Input: part model. Units: mm. Frame: model coordinates. Face numbers are marked on the shaded views. A direction names the side the tool comes from. Round coordinates to 2 decimals unless told otherwise and drop trailing zeros. Write each loop counter-clockwise with the first axis right and the second up, starting at its lowest first coordinate (ties: lowest second). Pieces come first, ordered by that corner, then holes. Notation, with made-up numbers: (76, -20) -> (91, -20) arc R22 ccw to (91, -2) -> close; hole circle Ø7 at (-25, 5.5). An arc over 180 degrees is marked (long way). Write item = value, one per line. Start each with the question number.
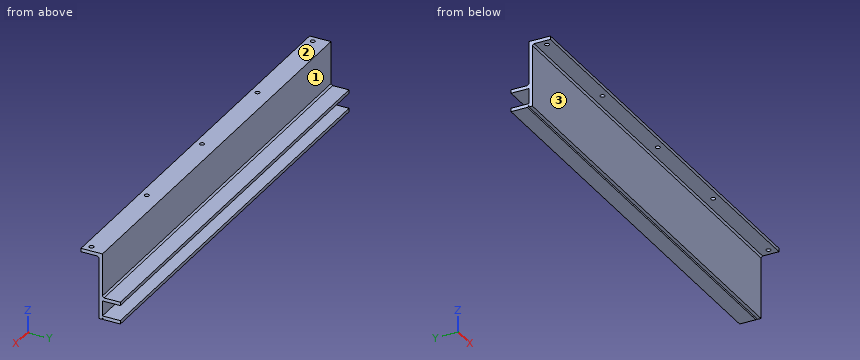
```python
from build123d import *

# Parameters (mm, degrees)
F0_W     = 609.6
F0_H     = 93.726
F1_DEPTH = 4.826
F3_DEPTH = 609.6
F5_D     = 6.35


with BuildPart() as f1:
    # F0 (on Front) → F1 (new body)
    with BuildSketch(Plane.XZ):
        Rectangle(F0_W, F0_H)
    extrude(amount=F1_DEPTH)

    # F2 (on face) → F3 (join, through all)
    with BuildSketch(Plane.YZ.offset(304.8)):
        Polygon((0, -13.335), (0, -15.621), (2.286, -15.621), align=None)
        Polygon((0, -15.621), (0, -20.447), (25.4, -20.447), (25.4, -15.621), (2.286, -15.621), align=None)
        Polygon((-30.226, 42.037), (-7.112, 42.037), (-4.826, 42.037), (-4.826, 46.863), (-30.226, 46.863), align=None)
        Polygon((0, -44.577), (2.286, -46.863), (25.4, -46.863), (25.4, -42.037), (0, -42.037), align=None)
        Polygon((-7.112, 42.037), (-4.826, 39.751), (-4.826, 42.037), align=None)
    extrude(amount=-F3_DEPTH)

    # F5 (through all)
    with Locations(Plane.XY.offset(46.863)):
        with Locations((-295.148, -20.574), (-147.574, -20.574), (0, -20.574), (147.574, -20.574), (295.148, -20.574)):
            Hole(F5_D / 2)


solid = f1.part
```
1. Section B-B (x = -126). Output: boundary loops of the cut face in (y, z) (3 decimals).
2. Pin query (flat end, axial travel): P1, Ø5, axis at x = 0, y = -20.574, coming from the +Z side; P2, Ø7.5, axis at x = -83.5, y = 9.5, coming from the +Z side; P3, Ø11, axis at x = 93, z = -29, coming from the +Y side; P4, Ø12, axis at x = 21.5, z = -5.5, coming from the -Y side. Return the tip coordinate at first contact, or that it passes through.
3. Line query: line 1 along Y through (x, z) = (0, 44); line 2 along Z through (x, y) = (80, 6); line 3 along Y through (x, z) = (220, -32). Output: solid intervals per line, ascending.
4. Reachability of the marked faces 1, 2 and 3 from +Z, -Z, +X, -X, +Y, -Y: full face, straight path, thin tool, end or side. Return the list, or none.
5. Section C-C (z = 12). Output: boundary loops of the cut face in (x, y).
6. Section A-A (y = 13.5). Output: boundary loops of the cut face in (x, z).
Check sheet entries:
q1.outline = (-30.226, 42.037) -> (-7.112, 42.037) -> (-4.826, 39.751) -> (-4.826, -46.863) -> (0, -46.863) -> (0, -44.577) -> (2.286, -46.863) -> (25.4, -46.863) -> (25.4, -42.037) -> (0, -42.037) -> (0, -20.447) -> (25.4, -20.447) -> (25.4, -15.621) -> (2.286, -15.621) -> (0, -13.335) -> (0, 46.863) -> (-30.226, 46.863) -> close
q2.P1 = through
q2.P2 = -15.62
q2.P3 = 0
q2.P4 = -4.83
q3.line_1 = -30.23 to -23.75, -17.4 to 0
q3.line_2 = -46.86 to -42.04, -20.45 to -15.62
q3.line_3 = -4.83 to 0
q4.face_1 = +Z, +X, -X, +Y
q4.face_2 = +Z, +X, -X, +Y, -Y
q4.face_3 = -Z, +X, -X, -Y
q5.outline = (-304.8, -4.83) -> (304.8, -4.83) -> (304.8, 0) -> (-304.8, 0) -> close
q6.outline = (-304.8, -46.86) -> (304.8, -46.86) -> (304.8, -42.04) -> (-304.8, -42.04) -> close; (-304.8, -20.45) -> (304.8, -20.45) -> (304.8, -15.62) -> (-304.8, -15.62) -> close
